Source: CAD feature listing. Evaluate the final solid. Frame: model axes, mm. Face numbers are marked on the shaded views. A direction names the side the tool comes from. Coordinates: 2 decimals unless noted, no trailing zeros. Order: outer loops, then holes, each group sorted by start corner. A loop starts at its lowest first (then second) coordinate and runs counter-clockwise, first axis right, second up. Notation, with made-up numbers: (-8.75, 83) -> (4.25, 83) arc R24 cw to (4.25, 99) -> close; hole circle Ø9 at (-3.5, 42.5). An arc over 180 degrees is marked (long way). Write each question's results on one line, items separated by ' | '. Start each with the question number.
from build123d import *

# Parameters (mm, degrees)
F0_W      = 75.59621
F0_H      = 14.2
F1_DEPTH  = 6
F3_DEPTH  = 14.2
F4_SIZE2  = 2
F4_SIZE   = 1
F5_SIZE2  = 5
F5_SIZE   = 5
F6_W      = 2
F6_H      = 8.2
F7_DEPTH  = 6
F9_DEPTH  = 2
F10_SIZE  = 0.5
F11_R     = 1.4
F12_DEPTH = 4


with BuildPart() as f1:
    # F0 (on Right) → F1 (new body)
    with BuildSketch(Plane.YZ):
        with Locations((-38.098105, 7.4)):
            Rectangle(F0_W, F0_H)
    extrude(amount=F1_DEPTH)

    # F2 (on face) → F3 (join, through all)
    with BuildSketch(Plane(origin=(0, 0, 0.3), x_dir=(1, 0, 0), z_dir=(0, 0, -1))):
        Polygon((0, 77.2236436599), (0, 75.89621), (6, 75.89621), align=None)
    extrude(amount=-F3_DEPTH)

    # F4
    f4_edges = [f1.edges().sort_by_distance(p)[0] for p in [
        (0, -38.761822, 0.3),
        (0, -38.761822, 14.5),
    ]]
    chamfer(f4_edges, length=F4_SIZE, length2=F4_SIZE2)

    # F5
    f5_edges = [f1.edges().sort_by_distance(p)[0] for p in [
        (0, -0.3, 7.4),
    ]]
    chamfer(f5_edges, length=F5_SIZE, length2=F5_SIZE2)

    # F6 (on face) → F7 (cut, through all)
    with BuildSketch(Plane(origin=(0, 0, 0), x_dir=(0, -1, 0), z_dir=(-1, 0, 0))):
        with Locations((42.2236436599, 7.4)):
            Rectangle(F6_W, F6_H)
        with Locations((66.2236436599, 7.4)):
            Rectangle(F6_W, F6_H)
        with Locations((46.2236436599, 7.4)):
            Rectangle(F6_W, F6_H)
        with Locations((50.2236436599, 7.4)):
            Rectangle(F6_W, F6_H)
        with Locations((54.2236436599, 7.4)):
            Rectangle(F6_W, F6_H)
        with Locations((58.2236436599, 7.4)):
            Rectangle(F6_W, F6_H)
        with Locations((62.2236436599, 7.4)):
            Rectangle(F6_W, F6_H)
    extrude(amount=-F7_DEPTH, mode=Mode.SUBTRACT)

    # F8 (on face) → F9 (cut)
    with BuildSketch(Plane(origin=(0, 0, 0), x_dir=(0, -1, 0), z_dir=(-1, 0, 0))):
        with BuildLine():
            Line((0.3, 3.25), (11.4, 3.25))
            ThreePointArc((11.4, 3.25), (15.55, 7.4), (11.4, 11.55))
            Line((11.4, 11.55), (0.3, 11.55))
            Line((0.3, 11.55), (0.3, 3.25))
        make_face()
    extrude(amount=-F9_DEPTH, mode=Mode.SUBTRACT)

    # F10
    f10_edges = [f1.edges().sort_by_distance(p)[0] for p in [
        (1, -4.3, 11.55),
        (0, -8.35, 11.55),
        (1, -4.3, 3.25),
    ]]
    chamfer(f10_edges, length=F10_SIZE)

    # F11 (on face) → F12 (cut, through all)
    with BuildSketch(Plane(origin=(2, 0, 0), x_dir=(0, -1, 0), z_dir=(-1, 0, 0))):
        with Locations((11.4, 7.4)):
            Circle(F11_R)
    extrude(amount=-F12_DEPTH, mode=Mode.SUBTRACT)


solid = f1.part
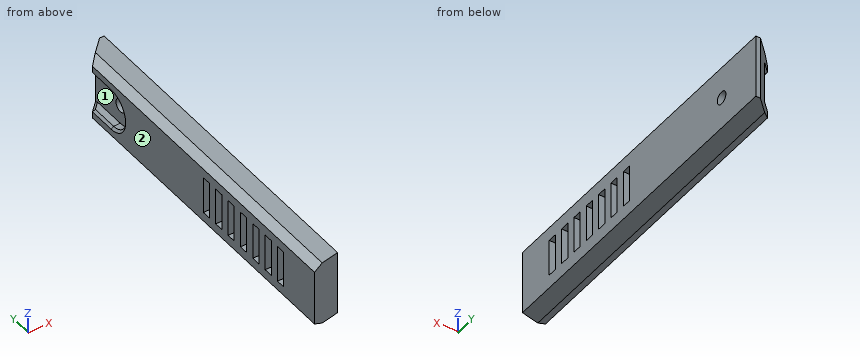
(1) Section A-A on x = 4.25. Count the separate pieces of the cut face and the enclosed holes in it, then the cut area to 3 significant figures.
(2) Reachability of the marked faces 1 and 2 from +Z, -Z, +X, -X, +Y, -Y: full face, straight path, thin tool, end or side. Return the list, or none.
(3) Section B-B on z = 2. Return the cut outline in (x, y), then the cut area to 3 significant figures.
(4) Line query: L1, parallel to Z at x = 4.55, y = -11.4; L2, parallel to X at y = -14, z = 4.75; L3, parallel to Y at x = 4.5, z = 1.5. Output: solid intervals per line, ascending.
(5) Section C-C on y = -30.5. Return the cut outline in (x, z), then the cut area to 3 significant figures.
(6) First-contact query: P1, Ø0.6, axis at x = 1.5, y = -62, coming from the -Z side; P2, Ø1.8, axis at x = 2, z = 8.5, coming from the -Y side; P3, Ø1.8, axis at x = 3, z = 8.5, coming from the -Y side. Flat tips, straight axial feed; report the tip coordinate or a pass-through.
Results list:
1) separate pieces: 1 | enclosed holes: 8 | area: 947 mm²
2) face 1: -X, +Y | face 2: +Z, -Z, -X, +Y, -Y
3) outline: (0, -77.22) -> (6, -75.9) -> (6, -0.3) -> (5, -0.3) -> (0, -5.3) -> close | area: 445 mm²
4) L1: z = 0.3 to 6, 8.8 to 14.5 | L2: x = 2 to 6 | L3: y = -76.23 to -0.8
5) outline: (0, 1.3) -> (2, 0.3) -> (6, 0.3) -> (6, 14.5) -> (2, 14.5) -> (0, 13.5) -> close | area: 83.2 mm²
6) P1: stops at z = 0.4 | P2: stops at y = -76.98 | P3: stops at y = -76.76
